from build123d import *

# Parameters (mm, degrees)
SKETCH1_W           = 90
SKETCH1_H           = 130
SKETCH1_W_2         = 10
SKETCH1_H_2         = 40
SKETCH1_W_3         = 40
SKETCH1_H_3         = 10
BOSS_EXTRUDE1_DEPTH = 5
SKETCH4_R           = 20
SKETCH4_R_2         = 15.5
BOSS_EXTRUDE2_DEPTH = 10


with BuildPart() as part:
    # Sketch1 → Boss-Extrude1 (new body)
    with BuildSketch(Plane(origin=(0, 0, 0), x_dir=(1, 0, 0), z_dir=(0, 1, 0))):
        with Locations((45, 65)):
            Rectangle(SKETCH1_W, SKETCH1_H)
        with Locations((-5, 65)):
            Rectangle(SKETCH1_W_2, SKETCH1_H_2)
        with Locations((95, 65)):
            Rectangle(SKETCH1_W_2, SKETCH1_H_2)
        with Locations((45, -5)):
            Rectangle(SKETCH1_W_3, SKETCH1_H_3)
        with Locations((45, 135)):
            Rectangle(SKETCH1_W_3, SKETCH1_H_3)
    extrude(amount=BOSS_EXTRUDE1_DEPTH)

    # Sketch4 → Boss-Extrude2 (add)
    with BuildSketch(Plane(origin=(0, 5, 0), x_dir=(1, 0, 0), z_dir=(0, 1, 0))):
        with Locations(Location((36.72, 31.47, 0), (0, 0, 270))):
            Circle(SKETCH4_R)
        with Locations(Location((36.72, 31.47, 0), (0, 0, 270))):
            Circle(SKETCH4_R_2, mode=Mode.SUBTRACT)
    extrude(amount=BOSS_EXTRUDE2_DEPTH)


solid = part.part
Input: part model. Units: mm. Frame: model coordinates. A direction names the side the tool comes from. Coordinates: 2 decimals unless noted, no trailing zeros. Loops run counter-clockwise (first coordinate to the right, second up) from the corner with the lowest first, then second, coordinate; pieces in that order, holes last.
Q1. Cut plane A-A (z = -31.47). Output: boundary loops of the cut face in (x, y).
Q2. Set-up query: faces 4 (the face through (77, 2, -130)), 5 (the face through (12, 2, 0)), 6 (the face through (77, 2, 0)). Return all of +Z, -Z, +X, -X, +Y, -Y with unobstructed straight access to the full face (end or side cutting, diameter ignored); none if empty.
Q3. Cut plane C-C (y = 13.25). Output: boundary loops of the cut face in (x, z), then the cut area to 3 significant figures.
Q4. Material intervals for line 1 (X direction, y = 8, z = -31.47); line 2 (Y direction, x = -2.5, z = -56.5); line 3 (Z direction, x = 44, y = 12.5), sorted ascending.
Q5. Draft query along X for faces 1 (the face through (45, 2, -140)), 2 (the face through (21.59, 9.93, -34.83)), 3 (the face through (-10, 2, -65)). Return one class per face: +X half, -X half, draft (parallel to the pull), parting line (faces both ways), or undercut.
Q6. Cut plane B-B (x = 36.72). Output: boundary loops of the cut face in (y, z), then the cut area to 3 significant figures.
Q7. Contact query for flat-ended pins moving along their axis: pin 1 (4 mm diameter, centred on y = 2.5, z = -103, fed in from +X); pin 2 (8 mm diameter, centred on x = 58.5, z = -111.5, fed in from -Y); pin 3 (4 mm diameter, centred on y = 1.5, z = -133.5, fed in from -X); pin 4 (1.5 mm diameter, centred on x = 7, y = 2, fed in from -Z). Output: stop coordinate, or through.
Q8. Cut plane D-D (x = 78.5). Output: boundary loops of the cut face in (y, z).
Working result:
1. outline: (0, 0) - (90, 0) - (90, 5) - (56.72, 5) - (56.72, 15) - (52.22, 15) - (52.22, 5) - (21.22, 5) - (21.22, 15) - (16.72, 15) - (16.72, 5) - (0, 5) - close
2. face 4: -Z, +X, +Y, -Y
2. face 5: +Z, -X, +Y, -Y
2. face 6: +Z, +X, +Y, -Y
3. outline: circle Ø40 at (36.72, -31.47); hole circle Ø31 at (36.72, -31.47)
3. area: 502 mm2
4. line 1: x = 16.72 to 21.22, 52.22 to 56.72
4. line 2: y = 0 to 5
4. line 3: z = -50.1 to -45.15, -17.79 to -12.84
5. face 1: draft
5. face 2: undercut
5. face 3: -X half
6. outline: (0, -140) - (5, -140) - (5, -51.47) - (15, -51.47) - (15, -46.97) - (5, -46.97) - (5, -15.97) - (15, -15.97) - (15, -11.47) - (5, -11.47) - (5, 10) - (0, 10) - close
6. area: 840 mm2
7. pin 1: stops at x = 90
7. pin 2: stops at y = 0
7. pin 3: stops at x = 25
7. pin 4: stops at z = -130
8. outline: (0, -130) - (5, -130) - (5, 0) - (0, 0) - close
